from build123d import *

# Parameters (mm, degrees)
SKETCH1_R           = 4.1
BOSS_EXTRUDE1_DEPTH = 2
SKETCH2_R           = 2
BOSS_EXTRUDE2_DEPTH = 5


with BuildPart() as part:
    # Sketch1 → Boss-Extrude1 (new body)
    with BuildSketch(Plane(origin=(0, 0, 0), x_dir=(1, 0, 0), z_dir=(0, 1, 0))):
        with BuildLine():
            Line((6.880964228, 1.749997239), (31.880964166, 1.749997239))
            ThreePointArc((31.880964166, 1.749997239), (36.598148239, 4.042144166), (37.711172654, 9.167272434))
            ThreePointArc((37.711172654, 9.167272434), (36.026057764, 14.43241452), (33.609947488, 19.40471223))
            ThreePointArc((33.609947488, 19.40471223), (34.250491945, 21.795256686), (36.641036401, 21.15471223))
            ThreePointArc((36.641036401, 21.15471223), (42.309424459, 0), (36.641036401, -21.15471223))
            ThreePointArc((36.641036401, -21.15471223), (34.250491945, -21.795256686), (33.609947488, -19.40471223))
            ThreePointArc((33.609947488, -19.40471223), (36.026056514, -14.432417639), (37.711171067, -9.167278965))
            ThreePointArc((37.711171067, -9.167278965), (36.598147218, -4.042150095), (31.880962823, -1.750002761))
            Line((31.880962823, -1.750002761), (6.880962823, -1.750002761))
            ThreePointArc((6.880962823, -1.750002761), (-0.000729594, -7.100011163), (-6.881322337, -1.748588554))
            Line((-6.881322337, -1.748588554), (-15.881322337, -1.748588554))
            ThreePointArc((-15.881322337, -1.748588554), (-16.588429118, -1.455695335), (-16.881322337, -0.748588554))
            Line((-16.881322337, -0.748588554), (-16.881322337, 0.748588554))
            ThreePointArc((-16.881322337, 0.748588554), (-16.588429118, 1.455695335), (-15.881322337, 1.748588554))
            Line((-15.881322337, 1.748588554), (-6.881322337, 1.748588554))
            ThreePointArc((-6.881322337, 1.748588554), (-0.000726746, 7.100011163), (6.880964228, 1.749997239))
        make_face()
        Circle(SKETCH1_R, mode=Mode.SUBTRACT)
    extrude(amount=BOSS_EXTRUDE1_DEPTH)

    # Sketch2 → Boss-Extrude2 (add)
    with BuildSketch(Plane(origin=(0, 2, 0), x_dir=(1, 0, 0), z_dir=(0, 1, 0))):
        with Locations((36.759322225, 17.141153462)):
            Circle(SKETCH2_R)
        with Locations((40.559424459, 0)):
            Circle(SKETCH2_R)
        with Locations((36.759322225, -17.141153462)):
            Circle(SKETCH2_R)
    extrude(amount=BOSS_EXTRUDE2_DEPTH)


solid = part.part
Can you work these out from the model? Positions are in its coordinate system, mm. A direction names the side the tool comes from. Give positions to 0.01 mm unless a question says otherwise; leave off trailing zeros. Loops run counter-clockwise (first coordinate to the right, second up) from the corner with the lowest first, then second, coordinate; pieces in that order, holes last. Notation, with made-up numbers: (86, 72) -> (91, 72) arc R21 ccw to (91, 94) -> close; hole circle Ø1 at (5.5, 51.25). An arc over 180 degrees is marked (long way). Return JSON: item names as keys, results as strings.
Q1. I want a section at B-B, the plane z = 0. List the corners of the cut face in (x, y) for me, then the cut area to 3 significant figures.
Checks:
{"outline": "(-16.88, 0) -> (-4.1, 0) -> (-4.1, 2) -> (-16.88, 2) -> close; (4.1, 0) -> (42.31, 0) -> (42.31, 2) -> (42.56, 2) -> (42.56, 7) -> (38.56, 7) -> (38.56, 2) -> (4.1, 2) -> close", "area": "122 mm2"}
Q2. I want a section at C-C, the plane y = 3.25. List the corners of the cut face in (x, z) for me.
Checks:
{"outline": "circle Ø4 at (36.76, -17.14); circle Ø4 at (36.76, 17.14); circle Ø4 at (40.56, 0)"}
Q3. I need wall thicknesses on probe 1 along X at (y, z) = (1.3, 0); probe 2 along Z at (x, y) = (0, 1.35); probe 3 along Y at (x, z) = (39, 11.5). Which ranges of each line are inside material? Lowest first, please.
Checks:
{"probe 1": "x = -16.88 to -4.1, 4.1 to 42.31", "probe 2": "z = -7.1 to -4.1, 4.1 to 7.1", "probe 3": "y = 0 to 2"}
Q4. On a 3-axis mill with a long thin cutter (end or side, diameter ignored), from which of +Z, -Z, +X, -X, +Y, -Y can I reach the whole of each face in a straight line? I mean faces 1 (the face through (-11, 1, -1.749)), 2 (the face through (36.55, 0.99, -3.98)), 3 (the face through (42.407, 4.465, 0.766)). Say none if no direction works.
Checks:
{"face 1": "-Z, -X, +Y, -Y", "face 2": "+Y, -Y", "face 3": "+Y"}
Q5. We'd pull the mould along Z, two halves only. Please class faces 4 (the face through (19, 1, -1.75)), 5 (the face through (38.61, 4.46, -16.38)), 6 (the face through (-11, 1, 1.749)): released by +Z, released by -Z, zero draft, split by the parting line, or undercut.
Checks:
{"face 4": "released by -Z", "face 5": "undercut", "face 6": "released by +Z"}
Q6. I want a section at A-A, the plane x = 0. List the corners of the cut face in (y, z) for me.
Checks:
{"outline": "(0, -7.1) -> (2, -7.1) -> (2, -4.1) -> (0, -4.1) -> close; (0, 4.1) -> (2, 4.1) -> (2, 7.1) -> (0, 7.1) -> close"}
Q7. For pin 1 Ø1 at (x, y) = (-11.5, 1) entering from -Z; pin 2 Ø1.4 at (x, z) = (35.5, -20) entering from +Y; pin 3 Ø0.9 at (x, z) = (38.5, 18) entering from -Y; pin 4 Ø0.6 at (x, y) = (-11.5, 1.5) entering from +Z, each with a flat end and sliding along its axis, tell me the tip position at first contact or that it passes through.
Checks:
{"pin 1": "stops at z = -1.75", "pin 2": "stops at y = 2", "pin 3": "stops at y = 0", "pin 4": "stops at z = 1.75"}
Q8. I want a section at D-D, the plane x = 17.5. List the corners of the cut face in (y, z) for me, then the cut area to 3 significant figures.
Checks:
{"outline": "(0, -1.75) -> (2, -1.75) -> (2, 1.75) -> (0, 1.75) -> close", "area": "7.00 mm2"}
